Verification items for the finished model (mm, model axes). A direction names the side the tool comes from. Give positions to 0.01 mm unless a question says otherwise; leave off trailing zeros. Write each loop counter-clockwise with the first axis right and the second up, starting at its lowest first coordinate (ties: lowest second). Pieces come first, ordered by that corner, then holes. Notation, with made-up numbers: M -38.75,47 L -20.75,47 A20 ccw -20.75,77 Z; hole C 28.5,46 d1. An arc over 180 degrees is marked long. Write item = value, one per line.
from build123d import *

# Parameters (mm, degrees)
SKETCH1_W                   = 96.1
SKETCH1_H                   = 96.1
SKETCH1_W_2                 = 80.1
SKETCH1_H_2                 = 80.1
BOSS_EXTRUDE1_DEPTH         = 6.35
FILLET1_R                   = 3
F_43_0_089_DIAMETER_HOLE1_D = 2.2606
F_43_0_089_DIAMETER_HOLE2_D = 2.2606


with BuildPart() as part:
    # Sketch1 → Boss-Extrude1 (new body)
    with BuildSketch(Plane(origin=(0, 0, 0), x_dir=(1, 0, 0), z_dir=(0, 1, 0))):
        Rectangle(SKETCH1_W, SKETCH1_H)
        Rectangle(SKETCH1_W_2, SKETCH1_H_2, mode=Mode.SUBTRACT)
    extrude(amount=BOSS_EXTRUDE1_DEPTH)

    # Fillet1
    fillet1_edges = [part.edges().sort_by_distance(p)[0] for p in [
        (-40.05, 3.175, 40.05),
        (40.05, 3.175, 40.05),
        (40.05, 3.175, -40.05),
        (-40.05, 3.175, -40.05),
        (-48.05, 3.175, -48.05),
        (48.05, 3.175, -48.05),
        (48.05, 3.175, 48.05),
        (-48.05, 3.175, 48.05),
    ]]
    fillet(fillet1_edges, radius=FILLET1_R)

    # #43 (0.089) Diameter Hole1 (through all)
    with Locations(Plane(origin=(0, 0, -48.05), x_dir=(-1, 0, 0), z_dir=(0, 0, -1))):
        with Locations((0, 3), (-37.55, 3), (37.55, 3)):
            Hole(F_43_0_089_DIAMETER_HOLE1_D / 2)

    # #43 (0.089) Diameter Hole2 (through all)
    with Locations(Plane.ZY.offset(48.05)):
        with Locations((0, 3), (-37.55, 3), (37.55, 3)):
            Hole(F_43_0_089_DIAMETER_HOLE2_D / 2)


solid = part.part
1) Depth check by flat-ended pin: P1, Ø2.5, axis at y = 3, z = -37.55, coming from the +X side; P2, Ø1.8, axis at y = 3, z = 0, coming from the +X side. Enter the tip coordinate at first touch or a pass-through.
From the geometry:
P1 = 48.05
P2 = through
2) Cross-section at D-D on y = 3. Count the separate pieces of the cut face and the enclosed holes in it, plus the area to 3 significant figures.
From the geometry:
separate_pieces = 12
enclosed_holes = 0
area = 2,600 mm^2
3) Cross-section at B-B on z = 6.5. Record the boundary of the cut face in (x, y), plus the area to 3 significant figures.
From the geometry:
outline = M -48.05,0 L -40.05,0 L -40.05,6.35 L -48.05,6.35 Z; M 40.05,0 L 48.05,0 L 48.05,6.35 L 40.05,6.35 Z
area = 102 mm^2
4) Material ranges on probe 1 along Z at (x, y) = (-44, 3.25); probe 2 along Z at (x, y) = (-11, 3.75), recorded low to high. Write a range as from..to.
From the geometry:
probe_1 = -48.05..-38.65, -36.45..-1.1, 1.1..36.45, 38.65..48.05
probe_2 = -48.05..-40.05, 40.05..48.05
5) Draft check along Z on faces 3 (the cylindrical face through (47.15, 3.22, 47.19)), 4 (the flat face through (40.05, 5, 1)), 5 (the cylindrical face through (47.15, 3.22, -47.19)), 6 (the flat face through (-43, 6.35, -1)). Enter one of: +Z half, -Z half, draft (parallel to the pull), parting line (faces both ways), or undercut.
From the geometry:
face_3 = +Z half
face_4 = undercut
face_5 = -Z half
face_6 = draft
6) Tool access check on faces 1 (the flat face through (-40.05, 5, 1)), 2 (the cylindrical face through (-38.68, 3.05, -43.75)). Record the directions out of +Z, -Z, +X, -X, +Y, -Y that give a thin tool (end or side, any length) a straight path to the whole face; none if there is none.
From the geometry:
face_1 = +Y, -Y
face_2 = +Z, -Z
7) Cross-section at A-A on x = 0. Record the boundary of the cut face in (y, z), plus the area to 3 significant figures.
From the geometry:
outline = M 0,-48.05 L 1.87,-48.05 L 1.87,-40.05 L 0,-40.05 Z; M 0,40.05 L 1.87,40.05 L 1.87,48.05 L 0,48.05 Z; M 4.13,-48.05 L 6.35,-48.05 L 6.35,-40.05 L 4.13,-40.05 Z; M 4.13,40.05 L 6.35,40.05 L 6.35,48.05 L 4.13,48.05 Z
area = 65.4 mm^2
8) Cross-section at C-C on x = 17. Record the boundary of the cut face in (y, z).
From the geometry:
outline = M 0,-48.05 L 6.35,-48.05 L 6.35,-40.05 L 0,-40.05 Z; M 0,40.05 L 6.35,40.05 L 6.35,48.05 L 0,48.05 Z
